The drawing under review shows one solid part. Ordinate dimensions are in mm from its lowest x, y, z. Round coordinates to 2 decimals unless told otherwise and drop trailing zeros. Order: outer loops, then holes, each group sorted by start corner. A loop starts at its lowest first (then second) coordinate and runs counter-clockwise, first axis right, second up. Notation, with made-up numbers: M 22.25,-8 L 46.25,-8 A22 cw 46.25,-1 Z; hole C 69,31.5 d5. An arc over 180 degrees is marked long. Answer as a JSON object with one key per item and string values. Group by question number.
1. Clearance check with a flat-ended pin moving along its axis: P1, Ø0.8, axis at y = 1.5, z = 256, coming from the -X side. State where the tip first meets the part, or that it passes through.
2. Add section B-B on z = 28. State the section outline as (x, y) points, and give its area (3 significant figures).
3. Add section A-A on y = 1.15. State the section outline as (x, z) points.
4. Add section C-C on z = 234.5. State the section outline as (x, y) points, and give its area (3 significant figures).
5. To check wall thickness, follow probe 1 along Z at (x, y) = (98, 1.85); probe 2 along X at (y, z) = (0.75, 199.5); probe 3 along X at (y, z) = (0.7, 90). State the ranges of each line that lie inside material, in increasing order. Write a range as [from, to].
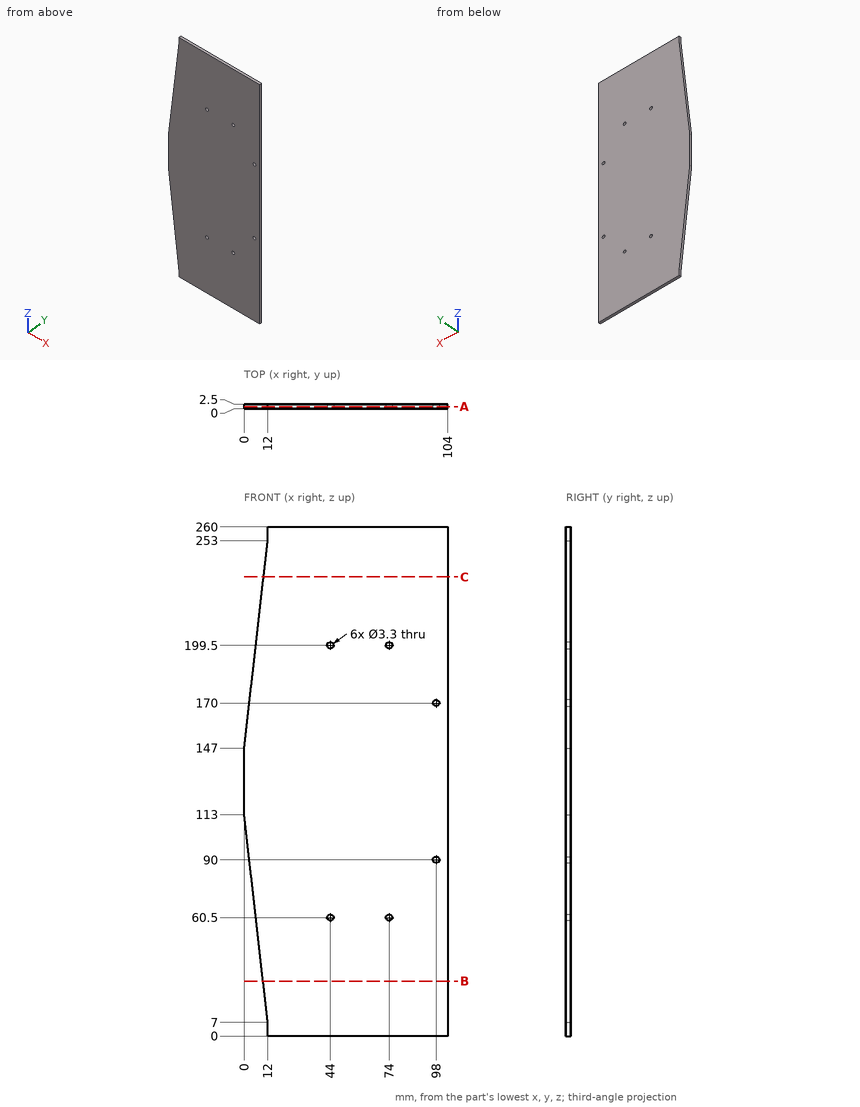
Recorded:
{
 "1": {"P1": "stops at x = 12"},
 "2": {"outline": "M 9.62,0 L 104,0 L 104,2.5 L 9.62,2.5 Z", "area": "236 mm²"},
 "3": {"outline": "M 0,113 L 12,7 L 12,0 L 104,0 L 104,260 L 12,260 L 12,253 L 0,147 Z; hole C 44,60.5 d3.3; hole C 44,199.5 d3.3; hole C 74,60.5 d3.3; hole C 74,199.5 d3.3; hole C 98,90 d3.3; hole C 98,170 d3.3"},
 "4": {"outline": "M 9.91,0 L 104,0 L 104,2.5 L 9.91,2.5 Z", "area": "235 mm²"},
 "5": {"probe 1": "z = [0, 88.35], [91.65, 168.35], [171.65, 260]", "probe 2": "x = [5.94, 42.35], [45.65, 72.35], [75.65, 104]", "probe 3": "x = [2.6, 96.35], [99.65, 104]"}
}
